Can you work these out from the model? Positions are in its coordinate system, mm. Face numbers are marked on the shaded views. A direction names the side the tool comes from. Give positions to 0.01 mm unless a question says otherwise; leave off trailing zeros. Order: outer loops, then holes, each group sorted by start corner. A loop starts at its lowest first (then second) coordinate and runs counter-clockwise, first axis right, second up. Notation, with made-up numbers: (9, -37.5) - (64, -37.5) arc R25 ccw to (64, -7.5) - close; hole circle Ø3 at (48.5, -10). An arc over 180 degrees is marked (long way). One line per question, with ' | ' between items.
Autodesk Inventor part; units mm, degrees
ref_plane "YZ Plane" through (0, 0, 0) normal (1, 0, 0) x (0, 1, 0)
ref_plane "XZ Plane" through (0, 0, 0) normal (0, 1, 0) x (-1, 0, 0)
ref_plane "XY Plane" through (0, 0, 0) normal (0, 0, 1) x (1, 0, 0)
sketch "Sketch1" plane through (0, 0, 0) normal (0, 0, 1) x (1, 0, 0)
  line L0 (0, 0) -> (13.97, 0)
  line L1 (13.97, 0) -> (13.97, 12.7)
  line L2 (13.97, 12.7) -> (0, 12.7)
  line L3 (0, 12.7) -> (0, 0)
  dimension "d0" = 13.97
  dimension "d1" = 12.7
extrude "Extrusion1" add sketch "Sketch1" along normal blind 6.35
sketch "Sketch2" plane through (0, 0, 0) normal (0, -1, 0) x (1, 0, 0)
  line L0 (0, 6.35) -> (13.97, 6.35)
  line L1 (0, 0) -> (13.97, 0)
  line L2 (3.81, 6.35) -> (10.16, 6.35)
  line L3 (10.16, 6.35) -> (10.16, 0)
  line L4 (10.16, 0) -> (3.81, 0)
  line L5 (3.81, 0) -> (3.81, 6.35)
  line L6 (0, 0) -> (0, 6.35)
  dimension "d4" = 6.35
  dimension "d5" = 3.81
extrude "Extrusion2" add sketch "Sketch2" along normal blind 6.35 contours L0 L3 L1 L5
properties part number "switchholder"
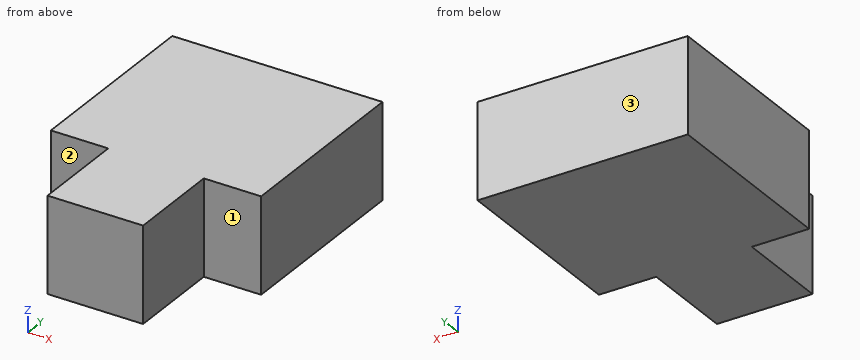
(1) Imagine slicing it at A-A (z = 2.5). List the corners of the cut face in (x, y) for me.
Answer below:
outline: (0, 0) - (3.81, 0) - (3.81, -6.35) - (10.16, -6.35) - (10.16, 0) - (13.97, 0) - (13.97, 12.7) - (0, 12.7) - close
(2) Imagine slicing it at B-B (x = 1.25). List the corners of the cut face in (y, z) for me.
Answer below:
outline: (0, 0) - (12.7, 0) - (12.7, 6.35) - (0, 6.35) - close
(3) Will these pins go through, and if not, where does the flat tip stop? pin 1 (3 mm diameter, centred on x = 13, z = 4, fed in from -Y); pin 2 (1 mm diameter, centred on y = -2, z = 4.5, fed in from +X); pin 3 (3 mm diameter, centred on y = -3, z = 2.5, fed in from -X).
Answer below:
pin 1: y = 0 | pin 2: x = 10.16 | pin 3: x = 3.81
(4) On a 3-axis mill with a long thin cutter (end or side, diameter ignored), from which of +Z, -Z, +X, -X, +Y, -Y can I reach the whole of each face in a straight line? I mean the marked faces 1, 2 and 3. Say none if no direction works.
Answer below:
face 1: +Z, -Z, +X, -Y | face 2: +Z, -Z, -X, -Y | face 3: +Z, -Z, +X, -X, +Y
(5) Imagine slicing it at C-C (y = -2). List the corners of the cut face in (x, z) for me.
Answer below:
outline: (3.81, 0) - (10.16, 0) - (10.16, 6.35) - (3.81, 6.35) - close
(6) If I drill on line 1 (X direction, y = -5.5, z = 1); line 2 (Y direction, x = 2.5, z = 3.75), over which ranges is the centre line in solid material (lowest first)?
Answer below:
line 1: 3.81 to 10.16 | line 2: 0 to 12.7
